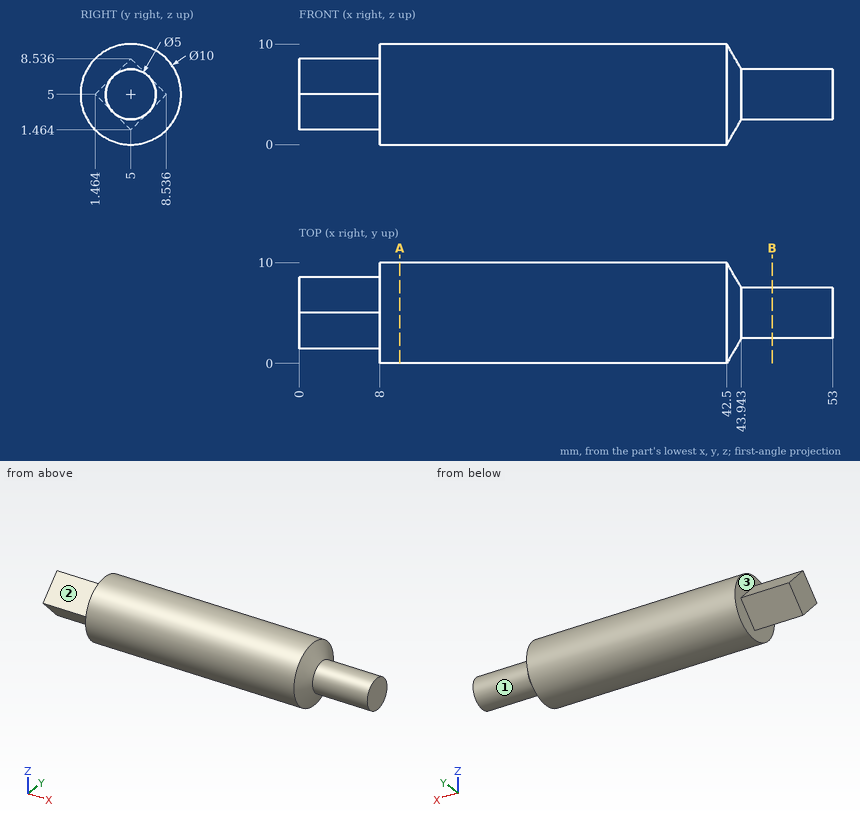
Geometry: see drawing. Coordinates: mm, zero at the bounding-box minimum. A direction names the side the tool comes from. Round coordinates to 2 decimals unless told otherwise and drop trailing zeros. Loops run counter-clockwise (first coordinate to the right, second up) from the corner with the lowest first, then second, coordinate; pieces in that order, holes last. Notation, with made-up numbers: (-18.5, 26.25) -> (11.5, 26.25) arc R16 cw to (11.5, 36.25) -> close; hole circle Ø1 at (5, 71). An arc over 180 degrees is marked (long way). Write each question's results on one line, items separated by ' | '.
1. Section A-A (x = 10). Return loops of the section in (y, z).
Geometry results:
outline: circle Ø10 at (5, 5)
2. Ray query, line 1 (Y direction, x = 31, z = 4.5) (1 decimal); line 2 (Y direction, x = 27, z = 9.5) (1 decimal); line 3 (Z direction, x = 23, y = 2.75) (1 decimal). Return the intervals inside material, ascending. Write a range as from..to.
Geometry results:
line 1: 0..10 | line 2: 2.8..7.2 | line 3: 0.5..9.5
3. First-contact query: P1, Ø1.5, axis at x = 22.5, y = 1, coming from the -Z side; P2, Ø4, axis at x = 13, z = 8, coming from the +Y side; P3, Ø3, axis at x = 30, z = 3, coming from the -Y side (1 decimal). Flat tips, straight axial feed; report the tip coordinate or a pass-through.
Geometry results:
P1: z = 1.2 | P2: y = 9.9 | P3: y = 0
4. Set-up query: the marked faces 1, 2 and 3. Return all of +Z, -Z, +X, -X, +Y, -Y with unobstructed straight access to the full face (end or side cutting, diameter ignored); none if empty.
Geometry results:
face 1: +X | face 2: +Z, -X, -Y | face 3: -X
5. Section B-B (x = 47). Return loops of the section in (y, z).
Geometry results:
outline: circle Ø5 at (5, 5)
